from build123d import *

# Parameters (mm, degrees)
ESBO_O1_R                  = 50
RESSALTO_EXTRUS_O1_DEPTH   = 2
ESBO_O2_R                  = 2.75
CORTE_EXTRUS_O1_DEPTH      = 2
CORTE_EXTRUS_O2_DEPTH      = 1
CORTE_EXTRUS_O2_DEPTH_BACK = 10
ESBO_O5_R                  = 1.5
ESBO_O5_R_2                = 1.75
CORTE_EXTRUS_O3_DEPTH      = 10


with BuildPart() as part:
    # Esboço1 → Ressalto-extrusão1 (new body)
    with BuildSketch(Plane.XY):
        Circle(ESBO_O1_R)
    extrude(amount=RESSALTO_EXTRUS_O1_DEPTH)

    # Esboço2 → Corte-extrusão1 (cut)
    with BuildSketch(Plane.XY.offset(2)):
        with Locations((-29, -34.409301068)):
            Circle(ESBO_O2_R)
        with Locations((29, -34.409301068)):
            Circle(ESBO_O2_R)
        with Locations((-38.824197531, 22.752619324)):
            Circle(ESBO_O2_R)
        with Locations((38.824197531, 22.752619324)):
            Circle(ESBO_O2_R)
    extrude(amount=-CORTE_EXTRUS_O1_DEPTH, mode=Mode.SUBTRACT)

    # Esboço4 → Corte-extrusão2 (cut, two sides)
    with BuildSketch(Plane.XY.offset(2)) as corte_extrus_o2_sk:
        Polygon((-40.723859979, -38.409301068), (44.57073926, -38.409301068), (1.923439641, -68.002213614), align=None)
    extrude(amount=CORTE_EXTRUS_O2_DEPTH, mode=Mode.SUBTRACT)
    extrude(corte_extrus_o2_sk.sketch, amount=-CORTE_EXTRUS_O2_DEPTH_BACK, mode=Mode.SUBTRACT)

    # Esboço5 → Corte-extrusão3 (cut)
    with BuildSketch(Plane(origin=(0, 0, 0), x_dir=(-1, 0, 0), z_dir=(0, 0, -1))):
        with Locations((5.1, 8.5)):
            Circle(ESBO_O5_R)
        with Locations((5.1, -12)):
            Circle(ESBO_O5_R)
        with Locations((-13.71, 23.86)):
            Circle(ESBO_O5_R_2)
        with Locations((13.29, 23.86)):
            Circle(ESBO_O5_R_2)
        with Locations((0, 42.87)):
            Circle(ESBO_O5_R_2)
    extrude(amount=-CORTE_EXTRUS_O3_DEPTH, mode=Mode.SUBTRACT)


solid = part.part
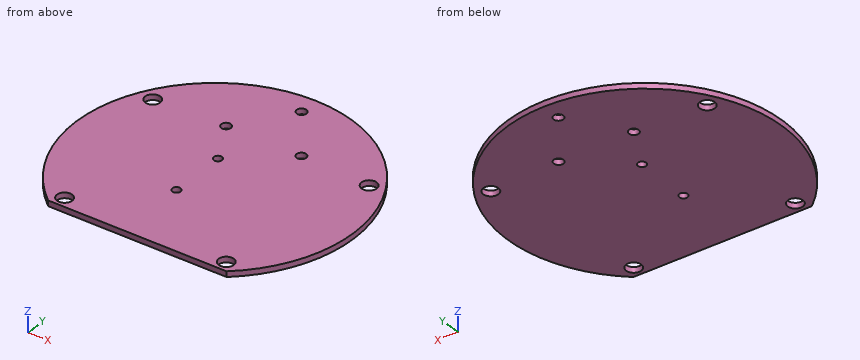
Input: part model. Units: mm. Frame: model coordinates. Round coordinates to 2 decimals unless told otherwise and drop trailing zeros. Order: outer loops, then holes, each group sorted by start corner. A loop starts at its lowest first (then second) coordinate and runs counter-clockwise, first axis right, second up. Notation, with made-up numbers: (38, -2.5) - (59, -2.5) arc R24 cw to (59, 12.5) - close; hole circle Ø1 at (15, 80.5). An arc over 180 degrees is marked (long way). Answer as a JSON object with one key per item and string values. Group by question number.
(1) Cut plane D-D (x = -25). Return loops of the section in (y, z).
(2) Material intervals for probe 1 along Y at (x, z) = (30.5, 1.6); probe 2 along Y at (x, z) = (-38, 1.4); probe 3 along Y at (x, z) = (-2, 1.1), sorted ascending. Write a range as from..to.
(3) Cut plane A-A (x = 0). Return loops of the section in (y, z), then the cut area to 3 significant figures.
(4) Cut plane B-B (y = 42.87). Return loops of the section in (x, z), then the cut area to 3 significant figures.
(5) Cut plane C-C (z = 1.5). Count the separate pieces of the cut face and the enclosed holes in it, then the cut area to 3 significant figures.
Here are the results:
{
 "1": {"outline": "(-38.41, 0) - (43.3, 0) - (43.3, 2) - (-38.41, 2) - close"},
 "2": {"probe 1": "y = -38.41..-36.71, -32.1..39.62", "probe 2": "y = -32.5..20.13, 25.38..32.5", "probe 3": "y = -38.41..49.96"},
 "3": {"outline": "(-38.41, 0) - (41.12, 0) - (41.12, 2) - (-38.41, 2) - close; (44.62, 0) - (50, 0) - (50, 2) - (44.62, 2) - close", "area": "170 mm^2"},
 "4": {"outline": "(-25.73, 0) - (-1.75, 0) - (-1.75, 2) - (-25.73, 2) - close; (1.75, 0) - (25.73, 0) - (25.73, 2) - (1.75, 2) - close", "area": "95.9 mm^2"},
 "5": {"separate pieces": "1", "enclosed holes": "9", "area": "7,210 mm^2"}
}
